from build123d import *

# Parameters (mm, degrees)
EXTRUDE_THIN1_DEPTH = 10


with BuildPart() as part:
    # Sketch1 → Extrude-Thin1 (new body)
    with BuildSketch(Plane(origin=(0, 0, 0), x_dir=(1, 0, 0), z_dir=(0, 1, 0))):
        with BuildLine():
            Line((-48.055213063, -4.381670713), (-48.055213063, -20.589409576))
            ThreePointArc((-48.055213063, -20.589409576), (-47.571938312, -21.756136971), (-46.405210296, -22.239410221))
            Line((-46.405210296, -22.239410221), (31.434177514, -22.239310121))
            ThreePointArc((31.434177514, -22.239310121), (32.600656469, -21.756281638), (33.08417589, -20.590006097))
            Line((33.08417589, -20.590006097), (33.103278784, 24.656648645))
            ThreePointArc((33.103278784, 24.656648645), (32.62001265, 25.824064412), (31.452603406, 26.307346307))
            Line((31.452603406, 26.307346307), (-29.991737035, 26.282239879))
            ThreePointArc((-29.991737035, 26.282239879), (-31.133079443, 25.823165706), (-31.639590763, 24.702068979))
            Line((-31.639590763, 24.702068979), (-31.602092863, 13.443859379))
            ThreePointArc((-31.602092863, 13.443859379), (-31.726631593, 12.809477673), (-32.0853545, 12.271641341))
            Line((-32.0853545, 12.271641341), (-47.571938464, -3.214942622))
            ThreePointArc((-47.571938464, -3.214942622), (-47.929614086, -3.75024202), (-48.055213063, -4.381670713))
        make_face()
        with BuildLine():
            Line((-46.055213063, -4.526644346), (-46.055213063, -20.239409771))
            Line((-46.055213063, -20.239409771), (31.084323774, -20.239310571))
            Line((31.084323774, -20.239310571), (31.103131072, 24.307203344))
            Line((31.103131072, 24.307203344), (-29.638181818, 24.282384176))
            Line((-29.638181818, 24.282384176), (-29.602103962, 13.4505225))
            ThreePointArc((-29.602103962, 13.4505225), (-29.877600157, 12.047189835), (-30.671140938, 10.857427779))
            Line((-30.671140938, 10.857427779), (-46.055213063, -4.526644346))
        make_face(mode=Mode.SUBTRACT)
    extrude(amount=EXTRUDE_THIN1_DEPTH)


solid = part.part
Here's how the part is built. I have some questions about the finished solid (model axes, mm). A direction names the side the tool comes from. Coordinates: 2 decimals unless noted, no trailing zeros. Order: outer loops, then holes, each group sorted by start corner. A loop starts at its lowest first (then second) coordinate and runs counter-clockwise, first axis right, second up. Notation, with made-up numbers: (28.5, -1.5) -> (80.5, -1.5) arc R22 cw to (80.5, 28.5) -> close; hole circle Ø5 at (-9, 16). An arc over 180 degrees is marked (long way). Answer in a Markdown table with one row per item.
(1) On a 3-axis mill with a long thin cutter (end or side, diameter ignored), from which of +Z, -Z, +X, -X, +Y, -Y can I reach the whole of each face in a straight line? I mean faces 5 (the face through (-2, 10, 21)), 6 (the face through (-29.87, 4.93, -12.07)). Say none if no direction works.
Answer key:
| item | result |
|---|---|
| face 5 | +Z, -Z, +X, -X, +Y |
| face 6 | +Y, -Y |
(2) Will these pins go through, and if not, where does the flat tip stop? pin 1 Ø2 at (x, y) = (-3, 8) entering from -Z; pin 2 Ø5 at (y, z) = (4.5, 3.5) entering from -X; pin 3 Ø5 at (y, z) = (3.5, 8) entering from +X.
Answer key:
| item | result |
|---|---|
| pin 1 | z = -26.29 |
| pin 2 | x = -48.06 |
| pin 3 | x = 33.09 |
(3) Thinking about a two-plate mould opening in X: for faces 1 (the face through (-39.72, 4.93, -4.637)), 2 (the face through (-38.26, 4.93, -3.27)), 3 (the face through (-2, 0, 21)), 4 (the face through (32.588, 4.93, 21.769)), which applies, +X half, -X half, draft (parallel to the pull), parting line (faces both ways), or undercut?
Answer key:
| item | result |
|---|---|
| face 1 | -X half |
| face 2 | undercut |
| face 3 | draft |
| face 4 | +X half |
(4) I want a section at C-C on x = -15. List the corners of the cut face in (y, z) for me, then the cut area to 3 significant figures.
Answer key:
| item | result |
|---|---|
| outline | (0, -26.29) -> (10, -26.29) -> (10, -24.29) -> (0, -24.29) -> close; (0, 20.24) -> (10, 20.24) -> (10, 22.24) -> (0, 22.24) -> close |
| area | 40.0 mm^2 |
(5) Please list where these lines run through material, in increasing order: probe 1 along Z at (x, y) = (15, 3); probe 2 along X at (y, z) = (3.75, 18); probe 3 along X at (y, z) = (9, -22).
Answer key:
| item | result |
|---|---|
| probe 1 | -26.3 to -24.3, 20.24 to 22.24 |
| probe 2 | -48.06 to -46.06, 31.09 to 33.09 |
| probe 3 | -31.63 to -29.63, 31.1 to 33.1 |
(6) I want a section at B-B on z = -4. List the corners of the cut face in (x, y) for me, then the cut area to 3 significant figures.
Answer key:
| item | result |
|---|---|
| outline | (-40.36, 0) -> (-37.53, 0) -> (-37.53, 10) -> (-40.36, 10) -> close; (31.09, 0) -> (33.09, 0) -> (33.09, 10) -> (31.09, 10) -> close |
| area | 48.3 mm^2 |
(7) I want a section at A-A on y = 3.5. List the corners of the cut face in (x, z) for me.
Answer key:
| item | result |
|---|---|
| outline | (-48.06, 4.38) arc R1.65 ccw to (-47.57, 3.21) -> (-32.09, -12.27) arc R1.65 cw to (-31.6, -13.44) -> (-31.64, -24.7) arc R1.65 ccw to (-29.99, -26.28) -> (31.45, -26.31) arc R1.65 ccw to (33.1, -24.66) -> (33.08, 20.59) arc R1.65 ccw to (31.43, 22.24) -> (-46.41, 22.24) arc R1.65 ccw to (-48.06, 20.59) -> close; hole (-46.06, 4.53) -> (-30.67, -10.86) arc R3.65 cw to (-29.6, -13.45) -> (-29.64, -24.28) -> (31.1, -24.31) -> (31.08, 20.24) -> (-46.06, 20.24) -> close |
